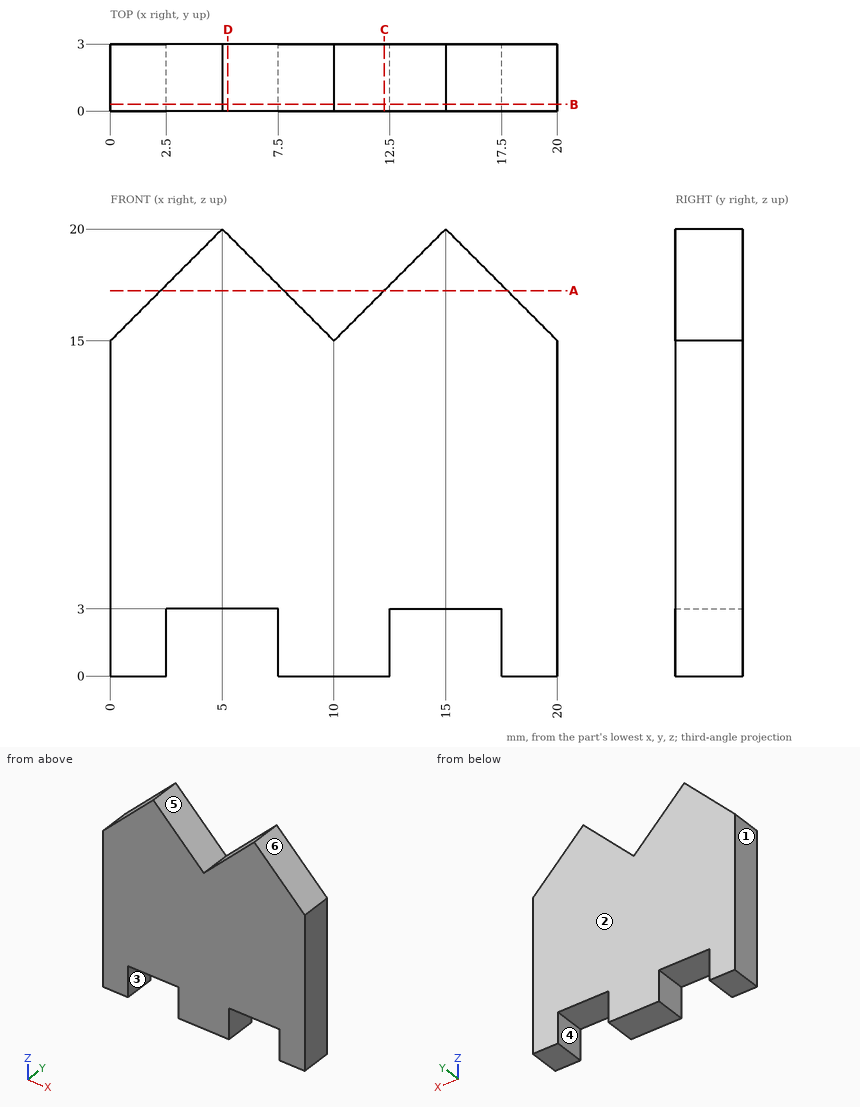
The drawing under review shows one solid part. Ordinate dimensions are in mm from its lowest x, y, z. A direction names the side the tool comes from. Give positions to 0.01 mm unless a question says otherwise; leave off trailing zeros. Write each loop counter-clockwise with the first axis right and the second up, starting at its lowest first coordinate (ties: lowest second). Pieces come first, ordered by that corner, then holes. Notation, with made-up numbers: (36, 8) - (64, 8) arc R19 ccw to (64, 43) - close; hole circle Ø11 at (28.25, 27). An arc over 180 degrees is marked (long way). Answer in a Markdown table with one row per item. Add a question column.
1. We need section B-B on y = 0.3. Write out the cut boundary in (x, z).
2. Tool access review of the marked faces 4, 5 and 6: name each direction out of +Z, -Z, +X, -X, +Y, -Y from which nothing blocks a thin tool from reaching the whole face with its end or side.
3. We need section D-D on x = 5.25. Write out the cut boundary in (y, z).
4. Wall thickness on line 1 along X through (y, z) = (1.85, 2); line 2 along X through (y, z) = (0.5, 18.5); line 3 along X through (y, z) = (1.55, 18): over which ranges is each line inside the solid? List them lowest first. Write a range as [from, to].
5. Draft analysis for pull direction X (two halves, no side actions). For the marked faces 1, 2 and 3, state which applies: +X half, -X half, draft (parallel to the pull), parting line (faces both ways), or undercut.
6. We need section C-C on x = 12.25. Write out the cut boundary in (y, z), then the cut area to 4 significant figures.
7. We need section A-A on z = 17.25. Write out the cut boundary in (x, y), then the cut area to 3 significant figures.
8. Insertion check: P1, Ø0.9, axis at x = 14, y = 1, coming from the -Z side. The pin has a flat end and moves straight along its axis. Give the tip position at first contact, or say it passes through.
Ans:
| question | item | result |
|---|---|---|
| 1 | outline | (0, 0) - (2.5, 0) - (2.5, 3) - (7.5, 3) - (7.5, 0) - (12.5, 0) - (12.5, 3) - (17.5, 3) - (17.5, 0) - (20, 0) - (20, 15) - (15, 20) - (10, 15) - (5, 20) - (0, 15) - close |
| 2 | face 4 | -Z, +Y, -Y |
| 2 | face 5 | +Z, +Y, -Y |
| 2 | face 6 | +Z, +X, +Y, -Y |
| 3 | outline | (0, 3) - (3, 3) - (3, 19.75) - (0, 19.75) - close |
| 4 | line 1 | x = [0, 2.5], [7.5, 12.5], [17.5, 20] |
| 4 | line 2 | x = [3.5, 6.5], [13.5, 16.5] |
| 4 | line 3 | x = [3, 7], [13, 17] |
| 5 | face 1 | -X half |
| 5 | face 2 | draft |
| 5 | face 3 | undercut |
| 6 | outline | (0, 0) - (3, 0) - (3, 17.25) - (0, 17.25) - close |
| 6 | area | 51.75 mm^2 |
| 7 | outline | (2.25, 0) - (7.75, 0) - (7.75, 3) - (2.25, 3) - close; (12.25, 0) - (17.75, 0) - (17.75, 3) - (12.25, 3) - close |
| 7 | area | 33.0 mm^2 |
| 8 | P1 | stops at z = 3 |
